from build123d import *

# Parameters (mm, degrees)
BOSS_EXTRUDE1_DEPTH   = 2.5
SKETCH3_W             = 0.65
SKETCH3_H             = 0.65
BOSS_EXTRUDE2_DEPTH   = 10
CHAMFER2_SIZE         = 0.15
CHAMFER2_SIZE2        = 0.259807621
CHAMFER3_SIZE         = 0.15
CHAMFER3_SIZE2        = 0.259807621
LPATTERN2_DEPTH       = 2.5
LPATTERN2_START       = -2.740192379
LPATTERN2_2_OUTLINE_W = 0.65
LPATTERN2_2_OUTLINE_H = 0.65
LPATTERN2_2_DEPTH     = 9.480384758


with BuildPart() as part:
    # Sketch1 → Boss-Extrude1 (new body)
    with BuildSketch(Plane(origin=(0, 0, 0), x_dir=(1, 0, 0), z_dir=(0, 1, 0))):
        Polygon((-7.42, 1.27), (-7.62, 1.07), (-7.62, -1.07), (-7.42, -1.27), (-5.28, -1.27), (-5.08, -1.07), (-5.08, 1.07), (-5.28, 1.27), align=None)
    extrude(amount=BOSS_EXTRUDE1_DEPTH)

    # Sketch3 → Boss-Extrude2 (add)
    with BuildSketch(Plane(origin=(0, -3, 0), x_dir=(1, 0, 0), z_dir=(0, 1, 0))):
        with Locations((-6.35, 0)):
            Rectangle(SKETCH3_W, SKETCH3_H)
    extrude(amount=BOSS_EXTRUDE2_DEPTH)

    # Chamfer2
    chamfer2_edges = [part.edges().sort_by_distance(p)[0] for p in [
        (-6.025, -3, 0),
        (-6.35, -3, -0.325),
        (-6.675, -3, 0),
        (-6.35, -3, 0.325),
    ]]
    chamfer2_side = [part.faces().sort_by_distance(p)[0] for p in [
        (-6.35, -3, 0),
    ]]
    chamfer(chamfer2_edges, length=CHAMFER2_SIZE, length2=CHAMFER2_SIZE2, reference=chamfer2_side[0])

    # Chamfer3
    chamfer3_edges = [part.edges().sort_by_distance(p)[0] for p in [
        (-6.025, 7, 0),
        (-6.35, 7, -0.325),
        (-6.675, 7, 0),
        (-6.35, 7, 0.325),
    ]]
    chamfer3_side = [part.faces().sort_by_distance(p)[0] for p in [
        (-6.35, 7, 0),
    ]]
    chamfer(chamfer3_edges, length=CHAMFER3_SIZE, length2=CHAMFER3_SIZE2, reference=chamfer3_side[0])

    # LPattern2: read off the stored shape, not the designer's step
    # LPattern2 outline → LPattern2 (add)
    with BuildSketch(Plane(origin=(0, 0, 0), x_dir=(1, 0, 0), z_dir=(0, 1, 0))):
        Polygon((-2.74, 1.27), (-4.88, 1.27), (-5.08, 1.07), (-5.08, -1.07), (-4.88, -1.27), (-2.74, -1.27), (-2.54, -1.07), (-2.34, -1.27), (-0.2, -1.27), (0, -1.07), (0.2, -1.27), (2.34, -1.27), (2.54, -1.07), (2.74, -1.27), (4.88, -1.27), (5.08, -1.07), (5.28, -1.27), (7.42, -1.27), (7.62, -1.07), (7.62, 1.07), (7.42, 1.27), (5.28, 1.27), (5.08, 1.07), (4.88, 1.27), (2.74, 1.27), (2.54, 1.07), (2.34, 1.27), (0.2, 1.27), (0, 1.07), (-0.2, 1.27), (-2.34, 1.27), (-2.54, 1.07), align=None)
    extrude(amount=LPATTERN2_DEPTH)

    # LPattern2 2 outline → LPattern2 2 (add)
    with BuildSketch(Plane(origin=(0, 0, 0), x_dir=(1, 0, 0), z_dir=(0, 1, 0)).offset(LPATTERN2_START)):
        with Locations((-3.81, 0)):
            Rectangle(LPATTERN2_2_OUTLINE_W, LPATTERN2_2_OUTLINE_H)
        with Locations((-1.27, 0)):
            Rectangle(LPATTERN2_2_OUTLINE_W, LPATTERN2_2_OUTLINE_H)
        with Locations((1.27, 0)):
            Rectangle(LPATTERN2_2_OUTLINE_W, LPATTERN2_2_OUTLINE_H)
        with Locations((3.81, 0)):
            Rectangle(LPATTERN2_2_OUTLINE_W, LPATTERN2_2_OUTLINE_H)
        with Locations((6.35, 0)):
            Rectangle(LPATTERN2_2_OUTLINE_W, LPATTERN2_2_OUTLINE_H)
    extrude(amount=LPATTERN2_2_DEPTH)

    # LPattern2 3: loft between two sections, ruled curve by curve
    lpattern2_3_from = [
        Edge.make_line((-3.985, -3, 0.175), (-3.635, -3, 0.175)),
        Edge.make_line((-3.635, -3, -0.175), (-3.985, -3, -0.175)),
        Edge.make_line((-3.635, -3, 0.175), (-3.635, -3, -0.175)),
        Edge.make_line((-3.985, -3, 0.175), (-3.985, -3, -0.175)),
    ]
    lpattern2_3_to = [
        Edge.make_line((-4.135, -2.740192379, 0.325), (-3.485, -2.740192379, 0.325)),
        Edge.make_line((-3.485, -2.740192379, -0.325), (-4.135, -2.740192379, -0.325)),
        Edge.make_line((-3.485, -2.740192379, 0.325), (-3.485, -2.740192379, -0.325)),
        Edge.make_line((-4.135, -2.740192379, 0.325), (-4.135, -2.740192379, -0.325)),
    ]
    lpattern2_3 = Solid(Shell([*[Face.make_surface_from_curves(lpattern2_3_from[k], lpattern2_3_to[k]) for k in range(4)], Face(Wire(lpattern2_3_from)), Face(Wire(lpattern2_3_to))]))
    add(lpattern2_3)

    # LPattern2 4: loft between two sections, ruled curve by curve
    lpattern2_4_from = [
        Edge.make_line((-1.445, -3, 0.175), (-1.095, -3, 0.175)),
        Edge.make_line((-1.095, -3, -0.175), (-1.445, -3, -0.175)),
        Edge.make_line((-1.095, -3, 0.175), (-1.095, -3, -0.175)),
        Edge.make_line((-1.445, -3, 0.175), (-1.445, -3, -0.175)),
    ]
    lpattern2_4_to = [
        Edge.make_line((-1.595, -2.740192379, 0.325), (-0.945, -2.740192379, 0.325)),
        Edge.make_line((-0.945, -2.740192379, -0.325), (-1.595, -2.740192379, -0.325)),
        Edge.make_line((-0.945, -2.740192379, 0.325), (-0.945, -2.740192379, -0.325)),
        Edge.make_line((-1.595, -2.740192379, 0.325), (-1.595, -2.740192379, -0.325)),
    ]
    lpattern2_4 = Solid(Shell([*[Face.make_surface_from_curves(lpattern2_4_from[k], lpattern2_4_to[k]) for k in range(4)], Face(Wire(lpattern2_4_from)), Face(Wire(lpattern2_4_to))]))
    add(lpattern2_4)

    # LPattern2 5: loft between two sections, ruled curve by curve
    lpattern2_5_from = [
        Edge.make_line((1.095, -3, 0.175), (1.445, -3, 0.175)),
        Edge.make_line((1.445, -3, -0.175), (1.095, -3, -0.175)),
        Edge.make_line((1.445, -3, 0.175), (1.445, -3, -0.175)),
        Edge.make_line((1.095, -3, 0.175), (1.095, -3, -0.175)),
    ]
    lpattern2_5_to = [
        Edge.make_line((0.945, -2.740192379, 0.325), (1.595, -2.740192379, 0.325)),
        Edge.make_line((1.595, -2.740192379, -0.325), (0.945, -2.740192379, -0.325)),
        Edge.make_line((1.595, -2.740192379, 0.325), (1.595, -2.740192379, -0.325)),
        Edge.make_line((0.945, -2.740192379, 0.325), (0.945, -2.740192379, -0.325)),
    ]
    lpattern2_5 = Solid(Shell([*[Face.make_surface_from_curves(lpattern2_5_from[k], lpattern2_5_to[k]) for k in range(4)], Face(Wire(lpattern2_5_from)), Face(Wire(lpattern2_5_to))]))
    add(lpattern2_5)

    # LPattern2 6: loft between two sections, ruled curve by curve
    lpattern2_6_from = [
        Edge.make_line((3.635, -3, 0.175), (3.985, -3, 0.175)),
        Edge.make_line((3.985, -3, -0.175), (3.635, -3, -0.175)),
        Edge.make_line((3.985, -3, 0.175), (3.985, -3, -0.175)),
        Edge.make_line((3.635, -3, 0.175), (3.635, -3, -0.175)),
    ]
    lpattern2_6_to = [
        Edge.make_line((3.485, -2.740192379, 0.325), (4.135, -2.740192379, 0.325)),
        Edge.make_line((4.135, -2.740192379, -0.325), (3.485, -2.740192379, -0.325)),
        Edge.make_line((4.135, -2.740192379, 0.325), (4.135, -2.740192379, -0.325)),
        Edge.make_line((3.485, -2.740192379, 0.325), (3.485, -2.740192379, -0.325)),
    ]
    lpattern2_6 = Solid(Shell([*[Face.make_surface_from_curves(lpattern2_6_from[k], lpattern2_6_to[k]) for k in range(4)], Face(Wire(lpattern2_6_from)), Face(Wire(lpattern2_6_to))]))
    add(lpattern2_6)

    # LPattern2 7: loft between two sections, ruled curve by curve
    lpattern2_7_from = [
        Edge.make_line((6.175, -3, 0.175), (6.525, -3, 0.175)),
        Edge.make_line((6.525, -3, -0.175), (6.175, -3, -0.175)),
        Edge.make_line((6.525, -3, 0.175), (6.525, -3, -0.175)),
        Edge.make_line((6.175, -3, 0.175), (6.175, -3, -0.175)),
    ]
    lpattern2_7_to = [
        Edge.make_line((6.025, -2.740192379, 0.325), (6.675, -2.740192379, 0.325)),
        Edge.make_line((6.675, -2.740192379, -0.325), (6.025, -2.740192379, -0.325)),
        Edge.make_line((6.675, -2.740192379, 0.325), (6.675, -2.740192379, -0.325)),
        Edge.make_line((6.025, -2.740192379, 0.325), (6.025, -2.740192379, -0.325)),
    ]
    lpattern2_7 = Solid(Shell([*[Face.make_surface_from_curves(lpattern2_7_from[k], lpattern2_7_to[k]) for k in range(4)], Face(Wire(lpattern2_7_from)), Face(Wire(lpattern2_7_to))]))
    add(lpattern2_7)

    # LPattern2 8: loft between two sections, ruled curve by curve
    lpattern2_8_from = [
        Edge.make_line((-3.485, 6.740192379, -0.325), (-4.135, 6.740192379, -0.325)),
        Edge.make_line((-4.135, 6.740192379, 0.325), (-3.485, 6.740192379, 0.325)),
        Edge.make_line((-4.135, 6.740192379, -0.325), (-4.135, 6.740192379, 0.325)),
        Edge.make_line((-3.485, 6.740192379, -0.325), (-3.485, 6.740192379, 0.325)),
    ]
    lpattern2_8_to = [
        Edge.make_line((-3.635, 7, -0.175), (-3.985, 7, -0.175)),
        Edge.make_line((-3.985, 7, 0.175), (-3.635, 7, 0.175)),
        Edge.make_line((-3.985, 7, -0.175), (-3.985, 7, 0.175)),
        Edge.make_line((-3.635, 7, -0.175), (-3.635, 7, 0.175)),
    ]
    lpattern2_8 = Solid(Shell([*[Face.make_surface_from_curves(lpattern2_8_from[k], lpattern2_8_to[k]) for k in range(4)], Face(Wire(lpattern2_8_from)), Face(Wire(lpattern2_8_to))]))
    add(lpattern2_8)

    # LPattern2 9: loft between two sections, ruled curve by curve
    lpattern2_9_from = [
        Edge.make_line((-0.945, 6.740192379, -0.325), (-1.595, 6.740192379, -0.325)),
        Edge.make_line((-1.595, 6.740192379, 0.325), (-0.945, 6.740192379, 0.325)),
        Edge.make_line((-1.595, 6.740192379, -0.325), (-1.595, 6.740192379, 0.325)),
        Edge.make_line((-0.945, 6.740192379, -0.325), (-0.945, 6.740192379, 0.325)),
    ]
    lpattern2_9_to = [
        Edge.make_line((-1.095, 7, -0.175), (-1.445, 7, -0.175)),
        Edge.make_line((-1.445, 7, 0.175), (-1.095, 7, 0.175)),
        Edge.make_line((-1.445, 7, -0.175), (-1.445, 7, 0.175)),
        Edge.make_line((-1.095, 7, -0.175), (-1.095, 7, 0.175)),
    ]
    lpattern2_9 = Solid(Shell([*[Face.make_surface_from_curves(lpattern2_9_from[k], lpattern2_9_to[k]) for k in range(4)], Face(Wire(lpattern2_9_from)), Face(Wire(lpattern2_9_to))]))
    add(lpattern2_9)

    # LPattern2 10: loft between two sections, ruled curve by curve
    lpattern2_10_from = [
        Edge.make_line((1.595, 6.740192379, -0.325), (0.945, 6.740192379, -0.325)),
        Edge.make_line((0.945, 6.740192379, 0.325), (1.595, 6.740192379, 0.325)),
        Edge.make_line((0.945, 6.740192379, -0.325), (0.945, 6.740192379, 0.325)),
        Edge.make_line((1.595, 6.740192379, -0.325), (1.595, 6.740192379, 0.325)),
    ]
    lpattern2_10_to = [
        Edge.make_line((1.445, 7, -0.175), (1.095, 7, -0.175)),
        Edge.make_line((1.095, 7, 0.175), (1.445, 7, 0.175)),
        Edge.make_line((1.095, 7, -0.175), (1.095, 7, 0.175)),
        Edge.make_line((1.445, 7, -0.175), (1.445, 7, 0.175)),
    ]
    lpattern2_10 = Solid(Shell([*[Face.make_surface_from_curves(lpattern2_10_from[k], lpattern2_10_to[k]) for k in range(4)], Face(Wire(lpattern2_10_from)), Face(Wire(lpattern2_10_to))]))
    add(lpattern2_10)

    # LPattern2 11: loft between two sections, ruled curve by curve
    lpattern2_11_from = [
        Edge.make_line((4.135, 6.740192379, -0.325), (3.485, 6.740192379, -0.325)),
        Edge.make_line((3.485, 6.740192379, 0.325), (4.135, 6.740192379, 0.325)),
        Edge.make_line((3.485, 6.740192379, -0.325), (3.485, 6.740192379, 0.325)),
        Edge.make_line((4.135, 6.740192379, -0.325), (4.135, 6.740192379, 0.325)),
    ]
    lpattern2_11_to = [
        Edge.make_line((3.985, 7, -0.175), (3.635, 7, -0.175)),
        Edge.make_line((3.635, 7, 0.175), (3.985, 7, 0.175)),
        Edge.make_line((3.635, 7, -0.175), (3.635, 7, 0.175)),
        Edge.make_line((3.985, 7, -0.175), (3.985, 7, 0.175)),
    ]
    lpattern2_11 = Solid(Shell([*[Face.make_surface_from_curves(lpattern2_11_from[k], lpattern2_11_to[k]) for k in range(4)], Face(Wire(lpattern2_11_from)), Face(Wire(lpattern2_11_to))]))
    add(lpattern2_11)

    # LPattern2 12: loft between two sections, ruled curve by curve
    lpattern2_12_from = [
        Edge.make_line((6.675, 6.740192379, -0.325), (6.025, 6.740192379, -0.325)),
        Edge.make_line((6.025, 6.740192379, 0.325), (6.675, 6.740192379, 0.325)),
        Edge.make_line((6.025, 6.740192379, -0.325), (6.025, 6.740192379, 0.325)),
        Edge.make_line((6.675, 6.740192379, -0.325), (6.675, 6.740192379, 0.325)),
    ]
    lpattern2_12_to = [
        Edge.make_line((6.525, 7, -0.175), (6.175, 7, -0.175)),
        Edge.make_line((6.175, 7, 0.175), (6.525, 7, 0.175)),
        Edge.make_line((6.175, 7, -0.175), (6.175, 7, 0.175)),
        Edge.make_line((6.525, 7, -0.175), (6.525, 7, 0.175)),
    ]
    lpattern2_12 = Solid(Shell([*[Face.make_surface_from_curves(lpattern2_12_from[k], lpattern2_12_to[k]) for k in range(4)], Face(Wire(lpattern2_12_from)), Face(Wire(lpattern2_12_to))]))
    add(lpattern2_12)


solid = part.part
The model under review builds one solid part; all positions refer to its coordinate system, in mm. Give positions to 0.01 mm unless a question says otherwise; leave off trailing zeros. Order: outer loops, then holes, each group sorted by start corner. A loop starts at its lowest first (then second) coordinate and runs counter-clockwise, first axis right, second up. Notation, with made-up numbers: M 71,26 L 98,26 A21 cw 98,49 Z; hole C 69.25,33 d2. An arc over 180 degrees is marked long. One line per question, with ' | ' between items. Start each with the question number.
1) Clearance check with flat-ended pins moving along their axes: P1, Ø1, axis at x = 5, z = -1, coming from the -Y side; P2, Ø0.7, axis at x = 3.5, y = -2, coming from the -Z side (3 decimals); P3, Ø0.5, axis at y = 5.5, z = 0, coming from the -X side (3 decimals); P4, Ø6, axis at x = -2.5, y = -2, coming from the -Z side. State where each tip first meets the part, or that it passes through.
2) Wall thickness on L1, parallel to X at y = -0.5, z = 0.15 (3 decimals); L2, parallel to Y at x = -4.5, z = -0.6; L3, parallel to Z at x = 6.5, y = -0.75 (3 decimals): over which ranges is each line inside the solid? List them lowest first. Write a range as from..to.
3) Consider section C-C, the plane z = 0.5. Give the boundary of the cut face in (x, y).
4) Consider section B-B, the plane x = 5.5. Give the boundary of the cut face in (y, z).
5) Consider section A-A, the plane y = 5.25. Give the boundary of the cut face in (x, z) (3 decimals).
6) Mouldability with a two-part tool opening along X and no side actions: class faces 1 (the face through (1, 1, -1.27)), 2 (the face through (0, 0, 0)), 3 (the face through (-7.62, 1, 0)) as pulls with the +X half, pulls with the -X half, needs draft (parallel to the pull), parting line crosses it, or undercut.
Found:
1) P1: stops at y = 0 | P2: stops at z = -0.325 | P3: stops at x = -6.675 | P4: stops at z = -1.27
2) L1: x = -6.675..-6.025, -4.135..-3.485, -1.595..-0.945, 0.945..1.595, 3.485..4.135, 6.025..6.675 | L2: y = 0..2.5 | L3: z = -0.325..0.325
3) outline: M -7.62,0 L 7.62,0 L 7.62,2.5 L -7.62,2.5 Z
4) outline: M 0,-1.27 L 2.5,-1.27 L 2.5,1.27 L 0,1.27 Z
5) outline: M -6.675,-0.325 L -6.025,-0.325 L -6.025,0.325 L -6.675,0.325 Z; M -4.135,-0.325 L -3.485,-0.325 L -3.485,0.325 L -4.135,0.325 Z; M -1.595,-0.325 L -0.945,-0.325 L -0.945,0.325 L -1.595,0.325 Z; M 0.945,-0.325 L 1.595,-0.325 L 1.595,0.325 L 0.945,0.325 Z; M 3.485,-0.325 L 4.135,-0.325 L 4.135,0.325 L 3.485,0.325 Z; M 6.025,-0.325 L 6.675,-0.325 L 6.675,0.325 L 6.025,0.325 Z
6) face 1: needs draft | face 2: undercut | face 3: pulls with the -X half
